```python
from build123d import *

# Parameters (mm, degrees)
F0_W           = 500
F0_H           = 150
F1_DEPTH       = 10
F2_D           = 4.5
F4_D           = 5.4
F4_CBORE_D     = 11.25
F4_CBORE_DEPTH = 6
F6_D           = 5


with BuildPart() as f1:
    # F0 (on Top) → F1 (new body)
    with BuildSketch(Plane.XY):
        Rectangle(F0_W, F0_H)
    extrude(amount=F1_DEPTH)

    # F2 (through all)
    with Locations(Plane(origin=(0, 0, 0), x_dir=(1, 0, 0), z_dir=(0, 0, -1))):
        with Locations((219.9761271477, -50), (159.9761271477, -50), (99.9761271477, -50), (39.9761271477, -50), (-20.0238728523, -50), (-80.0238728523, -50), (-140.0238728523, -50), (-200.0238728523, -50), (-200.0238728523, 50), (-140.0238728523, 50), (-80.0238728523, 50), (-20.0238728523, 50), (39.9761271477, 50), (99.9761271477, 50), (159.9761271477, 50), (219.9761271477, 50)):
            Hole(F2_D / 2)

    # F4 (through all)
    with Locations(Plane.XY.offset(10)):
        with Locations((200, 0), (150, 0), (100, 0), (50, 0), (0, 0), (-50, 0), (-100, 0), (-150, 0), (-200, 0)):
            CounterBoreHole(F4_D / 2, F4_CBORE_D / 2, F4_CBORE_DEPTH)

    # F6 (through all)
    with Locations(Plane.XY.offset(10)):
        with Locations((-233.4, 23), (-233.4, -23), (220, 23), (233, 23), (220, -23), (233, -23)):
            Hole(F6_D / 2)


solid = f1.part
```
Check sheet for the modelled part. Datum: model origin and axes. Units: mm. A direction names the side the tool comes from. Give positions to 0.01 mm unless a question says otherwise; leave off trailing zeros.
Item 1: Gauge pin test, flat end, axial feed: pin 1 (3.5 mm diameter, centred on x = -99, y = -2.5, fed in from +Z). Record the tip position at first contact, or that the pin passes through.
Item 2: Cross-section at A-A (z = 7). Count the separate pieces of the cut face and the enclosed holes in it, and give its area (3 significant figures).
Item 3: Access from +Z, -Z, +X, -X, +Y, -Y to the whole of each face (thin tool, end or side, straight path). Record for faces 4 (the face through (151, 3, 4)), 5 (the face through (-250, -1, 5)).
Item 4: Scan lines: L1, parallel to Y at x = -233.4, z = 5.5; L2, parallel to Y at x = 0, z = 6.3 (3 decimals); L3, parallel to Y at x = 158.5, z = 9. Record each from-to range of solid material in increasing order.
Item 5: Draft check along Y on faces 1 (the face through (205.365, 1.69, 7.042)), 2 (the face through (-94.635, 1.69, 7.042)), 3 (the face through (-3, 18, 10)). Enter one of: released by +Y, released by -Y, zero draft, split by the parting line, or undercut.
Report:
1. pin 1: stops at z = 4
2. separate pieces: 1
2. enclosed holes: 31
2. area: 73,700 mm2
3. face 4: +Z
3. face 5: +Z, -Z, -X, +Y, -Y
4. L1: y = -75 to -25.5, -20.5 to 20.5, 25.5 to 75
4. L2: y = -75 to -5.625, 5.625 to 75
4. L3: y = -75 to -51.7, -48.3 to 48.3, 51.7 to 75
5. face 1: undercut
5. face 2: undercut
5. face 3: zero draft
